Read the model definition and answer for the solid it produces. Units are mm, in the model's axes. Coordinates: 2 decimals unless noted, no trailing zeros. Loops run counter-clockwise (first coordinate to the right, second up) from the corner with the lowest first, then second, coordinate; pieces in that order, holes last.
from build123d import *

# Parameters (mm, degrees)
BOSS_EXTRUDE1_DEPTH      = 4
BOSS_EXTRUDE1_DEPTH_BACK = 4
SKETCH2_R                = 7.5
SKETCH2_R_2              = 10


with BuildPart() as part:
    # Sketch2 → Boss-Extrude1 (new, two sides: drawn at the far end of the back side and taken through both)
    with BuildSketch(Plane(origin=(0, 0, 0), x_dir=(0, 0, -1), z_dir=(1, 0, 0)).offset(-BOSS_EXTRUDE1_DEPTH_BACK)):
        with BuildLine():
            Line((-20, 0), (-20, -260))
            ThreePointArc((-20, -260), (0, -280), (20, -260))
            Line((20, -260), (20, 0))
            ThreePointArc((20, 0), (0, 20), (-20, 0))
        make_face()
        Circle(SKETCH2_R, mode=Mode.SUBTRACT)
        with Locations((0, -150)):
            Circle(SKETCH2_R_2, mode=Mode.SUBTRACT)
        with Locations((0, -260)):
            Circle(SKETCH2_R_2, mode=Mode.SUBTRACT)
    extrude(amount=BOSS_EXTRUDE1_DEPTH + BOSS_EXTRUDE1_DEPTH_BACK)


solid = part.part
Q1. A cutting plane is placed at A-A (y = -150). Give the vertices of the cut face in (x, z), then the cut area to 3 significant figures.
Findings below:
outline: (-4, -20) - (4, -20) - (4, -10) - (-4, -10) - close; (-4, 10) - (4, 10) - (4, 20) - (-4, 20) - close
area: 160 mm2
Q2. A cutting plane is placed at B-B (z = 0). Give the vertices of the cut face in (x, y), then the cut area to 3 significant figures.
Findings below:
outline: (-4, -280) - (4, -280) - (4, -270) - (-4, -270) - close; (-4, -250) - (4, -250) - (4, -160) - (-4, -160) - close; (-4, -140) - (4, -140) - (4, -7.5) - (-4, -7.5) - close; (-4, 7.5) - (4, 7.5) - (4, 20) - (-4, 20) - close
area: 1,960 mm2
Q3. Flat-ended cylindrical pins translate along their axes: pin 1 Ø4 at (x, z) = (1, -15.5) entering from -Y; pin 2 Ø1 at (x, z) = (-2, 0) entering from +Y. Find the tip coordinate at first contact, or state that the pin passes through.
Findings below:
pin 1: stops at y = -274.76
pin 2: stops at y = 20
Q4. Straight lines are drawn through the part: probe 1 along Y at (x, z) = (-2.25, 0); probe 2 along Y at (x, z) = (0.5, 9); probe 3 along Y at (x, z) = (-0.25, -4.5). For each, find the intervals that lie inside material, in ascending order.
Findings below:
probe 1: y = -280 to -270, -250 to -160, -140 to -7.5, 7.5 to 20
probe 2: y = -277.86 to -264.36, -255.64 to -154.36, -145.64 to 17.86
probe 3: y = -279.49 to -268.93, -251.07 to -158.93, -141.07 to -6, 6 to 19.49
Q5. A cutting plane is placed at C-C (x = -1.5). Give the vertices of the cut face in (y, z).
Findings below:
outline: (-260, -20) - (0, -20) arc R20 ccw to (0, 20) - (-260, 20) arc R20 ccw to start; hole circle Ø20 at (-260, 0); hole circle Ø20 at (-150, 0); hole circle Ø15 at (0, 0)
Q6. Determine the mould class of faces 1 (the face through (-0.056, -268.872, -4.614)), 2 (the face through (0, -132, -20)), 3 (the face through (-0.06, -159.76, 2.17)), 4 (the face through (0, 20, 0)) for opening direction Z: +Z half, -Z half, draft (parallel to the pull), parting line (faces both ways), or undercut.
Findings below:
face 1: undercut
face 2: -Z half
face 3: undercut
face 4: parting line
Q7. A cutting plane is placed at D-D (z = -17). Give the vertices of the cut face in (x, y).
Findings below:
outline: (-4, -270.54) - (4, -270.54) - (4, 10.54) - (-4, 10.54) - close
